Verification items for the finished model (mm, model axes). Face numbers are marked on the shaded views. A direction names the side the tool comes from. Coordinates: 2 decimals unless noted, no trailing zeros. Write each loop counter-clockwise with the first axis right and the second up, starting at its lowest first coordinate (ties: lowest second). Pieces come first, ordered by that corner, then holes. Notation, with made-up numbers: M 43,-20 L 100,-20 A30 cw 100,2 Z; hole C -8.75,53 d10. An arc over 180 degrees is marked long. One line per item, written item: value.
```python
from build123d import *

# Parameters (mm, degrees)
F0_R      = 17
F1_DEPTH  = 4
F2_R      = 2
F3_R      = 1.99999
F4_R      = 15
F4_R_2    = 2
F4_R_3    = 5.75
F5_DEPTH  = 0.25
F6_DEPTH  = 0.25
F7_R      = 11.5
F7_R_2    = 2
F7_R_3    = 5.75
F8_DEPTH  = 1
F9_R      = 11.5
F10_DEPTH = 1
F11_DEPTH = 5
F12_DEPTH = 0.5
F13_R     = 0.5
F14_DEPTH = 0.5
F13_R_2   = 2.5
F15_DEPTH = 2
F16_R     = 3
F17_DEPTH = 8.5
F18_R     = 1.5
F19_DEPTH = 9


# Not quite as in the source:
# - a fillet or chamfer is up to 0.001 mm smaller than in the source, because OpenCascade refuses the exact size


with BuildPart() as f1:
    # F0 (on Front) → F1 (new body)
    with BuildSketch(Plane.XZ):
        Circle(F0_R)
    extrude(amount=-F1_DEPTH)

    # F2
    f2_edges = [f1.edges().sort_by_distance(p)[0] for p in [
        (-17, 0, 0),
    ]]
    fillet(f2_edges, radius=F2_R)

    # F3 (radius 2 in the source; OpenCascade refuses exactly that, so slightly less here)
    f3_edges = [f1.edges().sort_by_distance(p)[0] for p in [
        (-17, 4, 0),
    ]]
    fillet(f3_edges, radius=F3_R)

    # F4 (on face) → F5 (cut)
    with BuildSketch(Plane.XZ):
        Circle(F4_R)
        with Locations((-6.1871843354, -6.1871843354)):
            Circle(F4_R_2, mode=Mode.SUBTRACT)
        with Locations((0, -8.75)):
            Circle(F4_R_2, mode=Mode.SUBTRACT)
        with Locations((6.1871843354, -6.1871843354)):
            Circle(F4_R_2, mode=Mode.SUBTRACT)
        with Locations((-8.75, 0)):
            Circle(F4_R_2, mode=Mode.SUBTRACT)
        with Locations((-6.1871843354, 6.1871843354)):
            Circle(F4_R_2, mode=Mode.SUBTRACT)
        Circle(F4_R_3, mode=Mode.SUBTRACT)
        with Locations((6.1871843354, 6.1871843354)):
            Circle(F4_R_2, mode=Mode.SUBTRACT)
        with Locations((8.75, 0)):
            Circle(F4_R_2, mode=Mode.SUBTRACT)
        with Locations((0, 8.75)):
            Circle(F4_R_2, mode=Mode.SUBTRACT)
    extrude(amount=-F5_DEPTH, mode=Mode.SUBTRACT)

    # F6 (cut): a face of the model
    f6_faces = [f1.faces().sort_by_distance(p)[0] for p in [
        (0, 4, 0),
    ]]
    extrude(f6_faces, amount=-F6_DEPTH, mode=Mode.SUBTRACT)

    # F7 (on face) → F8 (cut)
    with BuildSketch(Plane.XZ.offset(-0.25)):
        Circle(F7_R)
        with Locations((-6.1871843354, -6.1871843354)):
            Circle(F7_R_2, mode=Mode.SUBTRACT)
        with Locations((0, -8.75)):
            Circle(F7_R_2, mode=Mode.SUBTRACT)
        with Locations((6.1871843354, -6.1871843354)):
            Circle(F7_R_2, mode=Mode.SUBTRACT)
        with Locations((-8.75, 0)):
            Circle(F7_R_2, mode=Mode.SUBTRACT)
        with Locations((-6.1871843354, 6.1871843354)):
            Circle(F7_R_2, mode=Mode.SUBTRACT)
        Circle(F7_R_3, mode=Mode.SUBTRACT)
        with Locations((6.1871843354, 6.1871843354)):
            Circle(F7_R_2, mode=Mode.SUBTRACT)
        with Locations((8.75, 0)):
            Circle(F7_R_2, mode=Mode.SUBTRACT)
        with Locations((0, 8.75)):
            Circle(F7_R_2, mode=Mode.SUBTRACT)
    extrude(amount=-F8_DEPTH, mode=Mode.SUBTRACT)

    # F9 (on face) → F10 (cut)
    with BuildSketch(Plane(origin=(0, 3.75, 0), x_dir=(-1, 0, 0), z_dir=(0, 1, 0))):
        Circle(F9_R)
    extrude(amount=-F10_DEPTH, mode=Mode.SUBTRACT)

    # F11 (cut): faces of the model
    f11_faces = [f1.faces().sort_by_distance(p)[0] for p in [
        (8.75, 0, 0),
        (6.1871843354, 0, -6.1871843354),
        (0, 0, -8.75),
        (-8.75, 0, 0),
        (0, 0, 8.75),
        (6.1871843354, 0, 6.1871843354),
        (-6.1871843354, 0, -6.1871843354),
        (-6.1871843354, 0, 6.1871843354),
    ]]
    extrude(f11_faces, amount=-F11_DEPTH, mode=Mode.SUBTRACT)

    # F12 (cut): a face of the model
    f12_faces = [f1.faces().sort_by_distance(p)[0] for p in [
        (0, 0, 0),
    ]]
    extrude(f12_faces, amount=-F12_DEPTH, mode=Mode.SUBTRACT)

    # F13 (on face) → F14 (join)
    with BuildSketch(Plane.XZ.offset(-0.5)):
        with Locations((-2.2041946961, 3.0338137289)):
            Circle(F13_R)
        with Locations((-3.5664619361, 1.1588137289)):
            Circle(F13_R)
        with Locations((-3.5664619361, -1.1588137289)):
            Circle(F13_R)
        with Locations((-2.2041946961, -3.0338137289)):
            Circle(F13_R)
        with Locations((2.2041946961, -3.0338137289)):
            Circle(F13_R)
        with Locations((3.5664619361, -1.1588137289)):
            Circle(F13_R)
        with Locations((3.5664619361, 1.1588137289)):
            Circle(F13_R)
        with Locations((2.2041946961, 3.0338137289)):
            Circle(F13_R)
        with Locations((0, 3.75)):
            Circle(F13_R)
        with Locations((0, -3.75)):
            Circle(F13_R)
    extrude(amount=F14_DEPTH)

    # F13 (on face) → F15 (join)
    with BuildSketch(Plane.XZ.offset(-0.5)):
        Circle(F13_R_2)
    extrude(amount=F15_DEPTH)

    # F16 (on face) → F17 (join)
    with BuildSketch(Plane(origin=(0, 2.75, 0), x_dir=(-1, 0, 0), z_dir=(0, 1, 0))):
        Circle(F16_R)
    extrude(amount=F17_DEPTH)

    # F18 (on face) → F19 (cut)
    with BuildSketch(Plane(origin=(0, 11.25, 0), x_dir=(-1, 0, 0), z_dir=(0, 1, 0))):
        Circle(F18_R)
    extrude(amount=-F19_DEPTH, mode=Mode.SUBTRACT)


solid = f1.part
```
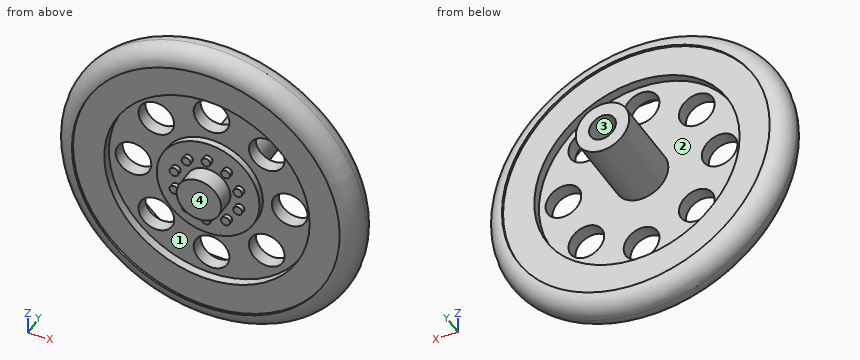
Item 1: Go/stop test with flat-tipped pins: P1, Ø4.5, axis at x = -8.75, z = 0, coming from the -Y side; P2, Ø3.5, axis at x = 6.19, z = 6.19, coming from the +Y side; P3, Ø1.5, axis at x = 4, z = -1.5, coming from the +Y side; P4, Ø1.1, axis at x = 2, z = -3, coming from the -Y side. Record where each tip stops, or that it passes through.
The answers:
P1: stops at y = 1.25
P2: passes through
P3: stops at y = 2.75
P4: stops at y = 0
Item 2: Access from +Z, -Z, +X, -X, +Y, -Y to the whole of each face (thin tool, end or side, straight path). Record for the marked faces 1 and 2.
The answers:
face 1: -Y
face 2: +Y
Item 3: Draft check along Z on the marked faces 3 and 4. Enter one of: released by +Z, released by -Z, zero draft, split by the parting line, or undercut.
The answers:
face 3: undercut
face 4: zero draft
Item 4: Cross-section at A-A, the plane y = 3.25. Enter the section's corners in (x, z), and give its area (3 significant figures).
The answers:
outline: C 0,0 d33.12; C 0,0 d6; hole C 0,0 d23; hole C 0,0 d3
area: 467 mm²
Item 5: Scan lines: line 1 (Z direction, x = 0, y = 0.85); line 2 (Y direction, x = 7, z = -2.5); line 3 (X direction, y = 2, z = -1.5). Record each from-to range of solid material in increasing order.
The answers:
line 1: z = -16.64 to -11.5, -5.75 to 5.75, 11.5 to 16.64
line 2: y = 1.25 to 2.75
line 3: x = -16.93 to -10.07, -7.43 to 7.43, 10.07 to 16.93
Item 6: Cross-section at B-B, the plane z = 0. Give the number of separate pieces and of enclosed holes in the cut face, and give its area (3 significant figures).
The answers:
separate pieces: 3
enclosed holes: 0
area: 102 mm²
